```python
from build123d import *

# Parameters (mm, degrees)
SKETCH1_W           = 20
SKETCH1_H           = 20
SKETCH1_R           = 5.1
BOSS_EXTRUDE2_DEPTH = 1.5
SKETCH1_4_W         = 60
SKETCH1_4_H         = 2
BOSS_EXTRUDE3_DEPTH = 20
FILLET1_R           = 3
FILLET2_R           = 3
FILLET3_R           = 3


with BuildPart() as part:
    # Sketch1 → Boss-Extrude2 (new body)
    with BuildSketch(Plane(origin=(0, 0, 0), x_dir=(1, 0, 0), z_dir=(0, 1, 0))):
        Rectangle(SKETCH1_W, SKETCH1_H)
        with Locations(Location((0, 0, 0), (0, 0, 270))):
            Circle(SKETCH1_R, mode=Mode.SUBTRACT)
    extrude(amount=BOSS_EXTRUDE2_DEPTH)

    # Sketch1_4 → Boss-Extrude3 (add)
    with BuildSketch(Plane(origin=(0, 0, 0), x_dir=(1, 0, 0), z_dir=(0, 1, 0))):
        with Locations((20, 11)):
            Rectangle(SKETCH1_4_W, SKETCH1_4_H)
    extrude(amount=BOSS_EXTRUDE3_DEPTH)

    # Fillet1
    fillet1_edges = [part.edges().sort_by_distance(p)[0] for p in [
        (0, 1.5, -10),
    ]]
    fillet(fillet1_edges, radius=FILLET1_R)

    # Fillet2
    fillet2_edges = [part.edges().sort_by_distance(p)[0] for p in [
        (10, 2.25, -10),
    ]]
    fillet(fillet2_edges, radius=FILLET2_R)

    # Fillet3
    fillet3_edges = [part.edges().sort_by_distance(p)[0] for p in [
        (10, 0.75, 10),
        (-10, 0.75, 10),
    ]]
    fillet(fillet3_edges, radius=FILLET3_R)


solid = part.part
```
Geometry: final body of the model. Coordinates: model frame, mm. A direction names the side the tool comes from. Round coordinates to 2 decimals unless told otherwise and drop trailing zeros. Loops run counter-clockwise (first coordinate to the right, second up) from the corner with the lowest first, then second, coordinate; pieces in that order, holes last. Notation, with made-up numbers: (-7.5, 82.5) -> (5.5, 82.5) arc R17 cw to (5.5, 97.5) -> close; hole circle Ø7 at (65, 49). An arc over 180 degrees is marked (long way). Use one line per item in the form item = value. Start each with the question number.
1) Access query for faces 4 (the flat face through (-2, 1.5, 5)), 5 (the flat face through (20, 10, -10)), 6 (the flat face through (10, 1, 0)). Directions: +Z, -Z, +X, -X, +Y, -Y. A direction counts if a zero-diameter tool reaches every point of the face in a straight line with its end or side. Return the directions, or none.
2) First-contact query: P1, Ø1.7, axis at y = 0.5, z = -3, coming from the +X side; P2, Ø1.5, axis at x = 13, y = 16.5, coming from the +Z side; P3, Ø8, axis at x = 10.5, y = 6, coming from the +Z side. Flat tips, straight axial feed; report the tip coordinate or a pass-through.
3) Section A-A on z = 0. Output: boundary loops of the cut face in (x, y), then the cut area to 3 significant figures.
4) Section D-D on x = 22. Output: boundary loops of the cut face in (y, z), then the cut area to 3 significant figures.
5) Draft query along X for faces 1 (the flat face through (20, 20, -11)), 2 (the cylindrical face through (1.532, 0.74, 4.864)), 3 (the cylindrical face through (-9.14, 0.76, 9.1)). Return one class per face: released by +X, released by -X, zero draft, split by the parting line, or undercut.
6) Section C-C on z = -3.25. Output: boundary loops of the cut face in (x, y), then the cut area to 3 significant figures.
7) Line query: L1, parallel to X at y = 0.6, z = 0; L2, parallel to Y at x = 1, z = 7.75; L3, parallel to Z at x = 30.5, y = 9.75. Output: solid intervals per line, ascending.
8) Section B-B on x = 0. Output: boundary loops of the cut face in (y, z).
Response:
q1.face_4 = +Z, +X, -X, +Y
q1.face_5 = +Z, +X, +Y
q1.face_6 = +Z, +X, +Y, -Y
q2.P1 = 10
q2.P2 = -10
q2.P3 = -8.66
q3.outline = (-10, 0) -> (-5.1, 0) -> (-5.1, 1.5) -> (-10, 1.5) -> close; (5.1, 0) -> (10, 0) -> (10, 1.5) -> (5.1, 1.5) -> close
q3.area = 14.7 mm^2
q4.outline = (0, -12) -> (20, -12) -> (20, -10) -> (0, -10) -> close
q4.area = 40.0 mm^2
q5.face_1 = zero draft
q5.face_2 = undercut
q5.face_3 = released by -X
q6.outline = (-10, 0) -> (-3.93, 0) -> (-3.93, 1.5) -> (-10, 1.5) -> close; (3.93, 0) -> (10, 0) -> (10, 1.5) -> (3.93, 1.5) -> close
q6.area = 18.2 mm^2
q7.L1 = -10 to -5.1, 5.1 to 10
q7.L2 = 0 to 1.5
q7.L3 = -12 to -10
q8.outline = (0, -12) -> (20, -12) -> (20, -10) -> (4.5, -10) arc R3 cw to (1.5, -7) -> (1.5, -5.1) -> (0, -5.1) -> close; (0, 5.1) -> (1.5, 5.1) -> (1.5, 10) -> (0, 10) -> close
